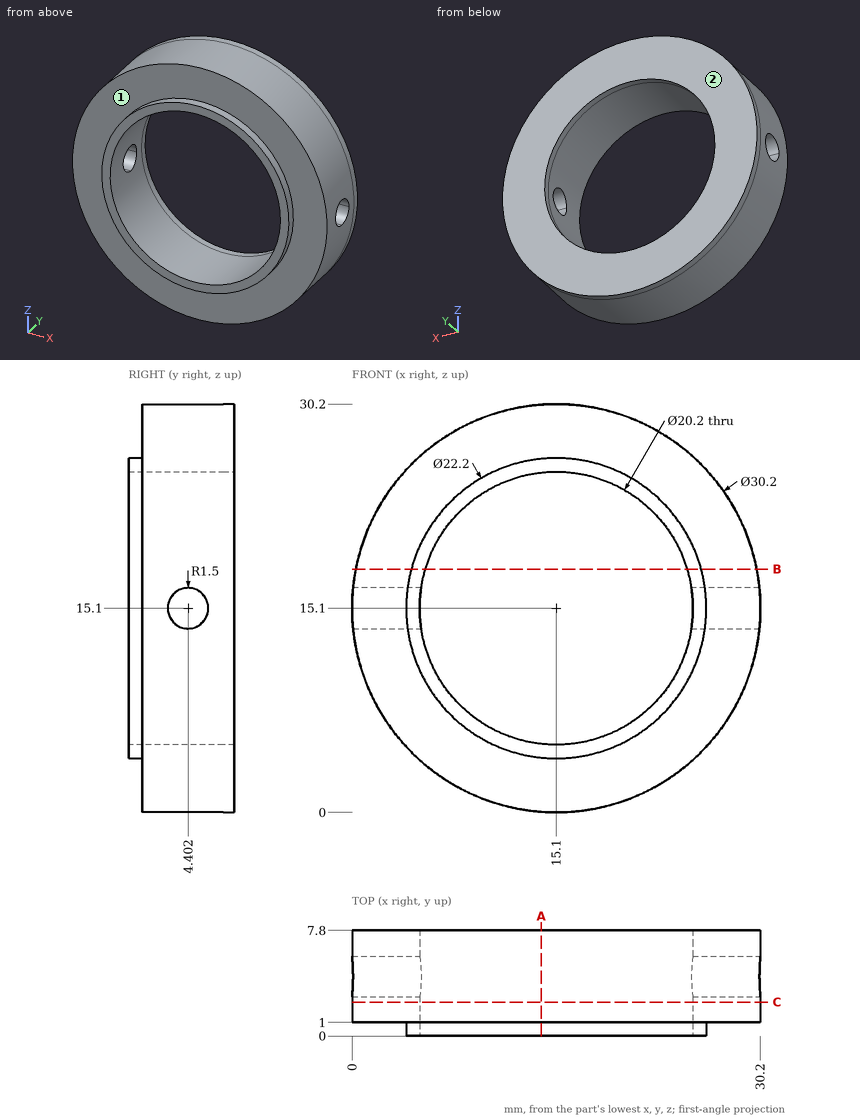
Part print with two shaded views. Sizes in mm from the minimum x, y, z corner. A direction names the side the tool comes from. Give positions to 0.01 mm unless a question says otherwise; leave off trailing zeros. Order: outer loops, then holes, each group sorted by start corner. A loop starts at its lowest first (then second) coordinate and runs counter-clockwise, first axis right, second up.
1) Saw through at B-B, the plane z = 18. Write the cut outline in (x, y).
2) Saw through at C-C, the plane y = 2.5. Write the cut outline in (x, z).
3) Pin check, flat tips, straight feed: pin 1 (3 mm diameter, centred on x = 5.5, y = 6.5, fed in from +Z); pin 2 (4 mm diameter, centred on y = 3, z = 27, fed in from +X); pin 3 (1 mm diameter, centred on y = 7, z = 14, fed in from +X). Stop position of each tip, or through.
4) 3-axis set-ups, long thin cutter, end or side, ignore diameter. For the marked faces 1 and 2: which of +Z, -Z, +X, -X, +Y, -Y reach the whole face in a straight line?
5) Wall check: probe 1 along Y at (x, z) = (29, 13); probe 2 along Y at (x, z) = (28, 16); probe 3 along Z at (x, y) = (13.5, 3) (1 decimal). Give the ranges that are in metal, low to high.
6) Saw through at A-A, the plane x = 14. Write the cut outline in (y, z), then the cut area to 3 significant figures.
Computed:
1. outline: (0.28, 1) - (4.39, 1) - (4.39, 0) - (5.43, 0) - (5.43, 7.8) - (0.28, 7.8) - close; (24.77, 0) - (25.81, 0) - (25.81, 1) - (29.92, 1) - (29.92, 7.8) - (24.77, 7.8) - close
2. outline: circle Ø30.2 at (15.1, 15.1); hole circle Ø20.2 at (15.1, 15.1)
3. pin 1: stops at z = 27.84
3. pin 2: stops at x = 26.5
3. pin 3: stops at x = 30.19
4. face 1: -Y
4. face 2: +Z, -Z, +X, -X, +Y
5. probe 1: y = 1 to 7.8
5. probe 2: y = 1 to 3.2, 5.6 to 7.8
5. probe 3: z = 0.1 to 5.1, 25.1 to 30.1
6. outline: (0, 4.05) - (1, 4.05) - (1, 0.04) - (7.8, 0.04) - (7.8, 5.06) - (0, 5.06) - close; (0, 25.14) - (7.8, 25.14) - (7.8, 30.16) - (1, 30.16) - (1, 26.15) - (0, 26.15) - close
6. area: 70.3 mm2
